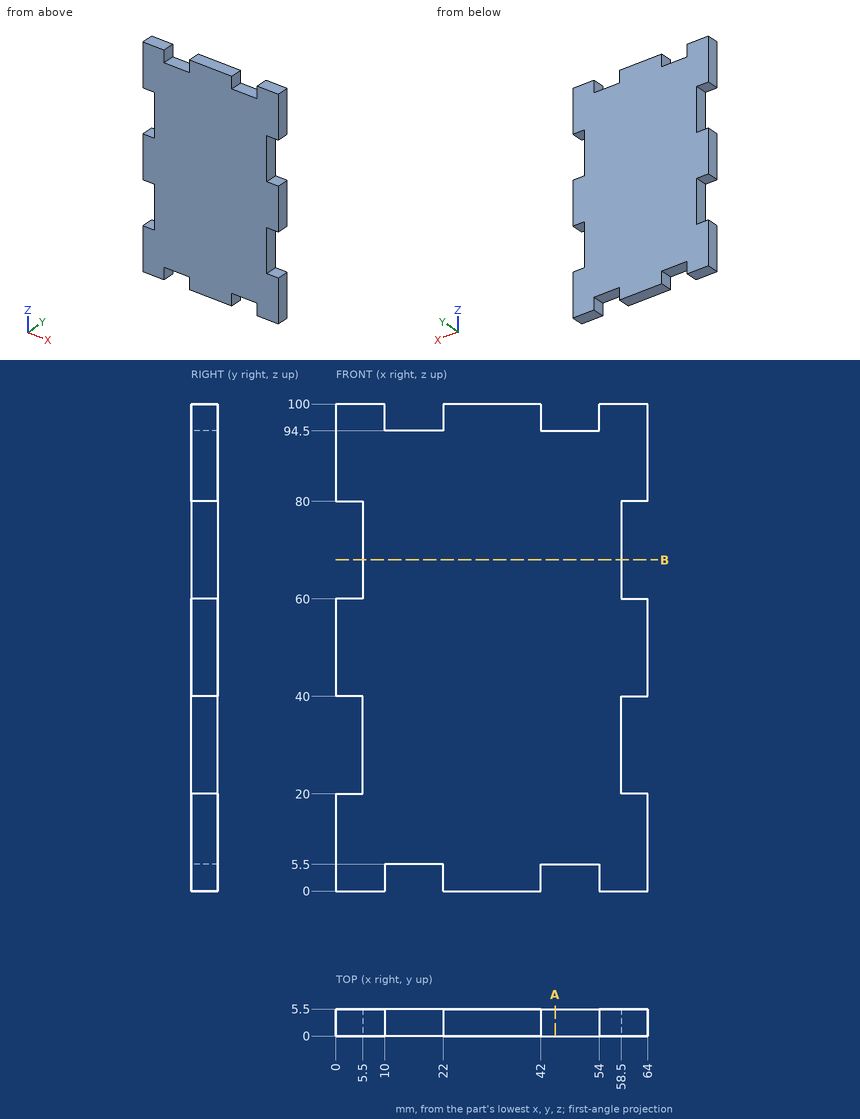
Can you work these out from the drawing? Everything is in mm from the part's minimum corner. Coordinates: 2 decimals unless noted, no trailing zeros. Loops run counter-clockwise (first coordinate to the right, second up) from the corner with the lowest first, then second, coordinate; pieces in that order, holes last.
1. For P1, Ø1, axis at y = 3.5, z = 67, coming from the +X side; P2, Ø3, axis at x = 14.5, y = 2, coming from the +Z side; P3, Ø2, axis at x = 49.5, y = 3.5, coming from the -Z side, each with a flat end and sliding along its axis, tell me the tip position at first contact or that it passes through.
2. Imagine slicing it at A-A, the plane x = 45. Please give me the cut outline in (y, z), and give its area (4 significant figures).
3. Imagine slicing it at B-B, the plane z = 68. Please give me the cut outline in (x, y).
4. I need wall thicknesses on L1, parallel to Z at x = 60, y = 1.4; L2, parallel to X at y = 2.4, z = 30; L3, parallel to Z at x = 51, y = 0.35. Which ranges of each line are inside material? Lowest first, please.
Taken from the geometry:
1. P1: stops at x = 58.5
1. P2: stops at z = 94.5
1. P3: stops at z = 5.5
2. outline: (0, 5.5) - (5.5, 5.5) - (5.5, 94.5) - (0, 94.5) - close
2. area: 489.5 mm2
3. outline: (5.5, 0) - (58.5, 0) - (58.5, 5.5) - (5.5, 5.5) - close
4. L1: z = 0 to 20, 40 to 60, 80 to 100
4. L2: x = 5.5 to 58.5
4. L3: z = 5.5 to 94.5
